from build123d import *

# Parameters (mm, degrees)
BOSS_EXTRU_1_DEPTH      = 6
ESQUISSE4_R             = 1.55
ENL_V_MAT_EXTRU_3_DEPTH = 6


with BuildPart() as part:
    # Esquisse3 → Boss.-Extru.1 (new body)
    with BuildSketch(Plane.XY):
        with BuildLine():
            Line((-7, -132), (-7, 58))
            ThreePointArc((-7, 58), (-2, 63), (3, 58))
            Line((3, 58), (3, -132))
            ThreePointArc((3, -132), (-2, -137), (-7, -132))
        make_face()
    extrude(amount=BOSS_EXTRU_1_DEPTH)

    # Esquisse4 → Enlèv. mat.-Extru.3 (cut)
    with BuildSketch(Plane(origin=(0, 0, 0), x_dir=(-1, 0, 0), z_dir=(0, 0, -1))):
        with Locations((2, -127)):
            Circle(ESQUISSE4_R)
        with Locations(Location((2, 58, 0), (0, 0, 180))):
            Circle(ESQUISSE4_R)
    extrude(amount=-ENL_V_MAT_EXTRU_3_DEPTH, mode=Mode.SUBTRACT)


solid = part.part
Build history of the part. All positions in model axes, mm. Coordinates: 2 decimals unless noted, no trailing zeros. Order: outer loops, then holes, each group sorted by start corner. A loop starts at its lowest first (then second) coordinate and runs counter-clockwise, first axis right, second up. Notation, with made-up numbers: (70.5, 61) - (105.5, 61) arc R24 cw to (105.5, 85) - close; hole circle Ø8 at (66, 85). An arc over 180 degrees is marked (long way). Write item = value, one per line. Start each with the question number.
1) Two-plate mould, pull along X, no slides. Class faces 1 (the face through (-2, -137, 3)), 2 (the face through (-7, -38, 3)), 3 (the face through (-2.202, 56.463, 2.958)): pulls with the +X half, pulls with the -X half, needs draft (parallel to the pull), parting line crosses it, or undercut.
2) Wall check: line 1 along Y through (x, z) = (-2, 1.85); line 2 along X through (y, z) = (-127, 3.15); line 3 along Y through (x, z) = (2, 5.4). Give the ranges that are in metal, low to high. Write a range as from..to.
3) Flat gauge pins, fed straight in: pin 1 Ø3 at (x, y) = (-2, -127) entering from -Z; pin 2 Ø1.5 at (x, z) = (-5, 3.5) entering from -Y. Where does each tip first touch, or does it go through?
4) Saw through at B-B on z = 4.3. Write the cut outline in (x, y), then the cut area to 3 significant figures.
5) Saw through at A-A on x = -2. Write the cut outline in (y, z).
From the geometry:
q1.face_1 = parting line crosses it
q1.face_2 = pulls with the -X half
q1.face_3 = undercut
q2.line_1 = -137..-128.55, -125.45..56.45, 59.55..63
q2.line_2 = -7..-3.55, -0.45..3
q2.line_3 = -135..61
q3.pin_1 = through
q3.pin_2 = -136.47
q4.outline = (-7, -132) arc R5 ccw to (3, -132) - (3, 58) arc R5 ccw to (-7, 58) - close; hole circle Ø3.1 at (-2, -127); hole circle Ø3.1 at (-2, 58)
q4.area = 1,960 mm^2
q5.outline = (-137, 0) - (-128.55, 0) - (-128.55, 6) - (-137, 6) - close; (-125.45, 0) - (56.45, 0) - (56.45, 6) - (-125.45, 6) - close; (59.55, 0) - (63, 0) - (63, 6) - (59.55, 6) - close
